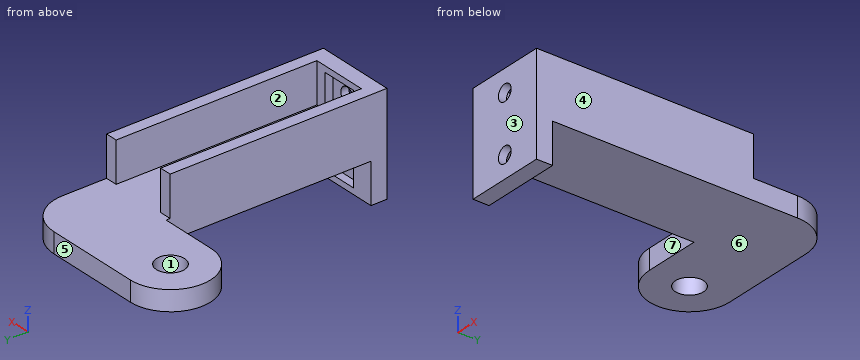
```python
from build123d import *

# Parameters (mm, degrees)
SKETCH1_R          = 1.75
AXLEHOLDER_DEPTH   = 2.5
SKETCH1_3_W        = 10
SKETCH1_3_H        = 2
BASE_DEPTH         = 7.5
BASE_DEPTH_BACK    = 5
SKETCH2_R          = 1
BOLTHOLES_DEPTH    = 3
SKETCH3_W          = 4.5
SKETCH3_H          = 4
NUTSLOTS_DEPTH     = 1
SKETCH4_W          = 1.5
SKETCH4_H          = 5
STIFFENERRIB_DEPTH = 25


with BuildPart() as part:
    # Sketch1 → AxleHolder (new body)
    with BuildSketch(Plane.XY):
        with BuildLine():
            Line((-12, 27.5), (-5, 27.5))
            Line((-5, 27.5), (-5, 0))
            Line((-5, 0), (5, 0))
            Line((5, 0), (5, 32.5))
            ThreePointArc((5, 32.5), (3.535533906, 36.035533906), (0, 37.5))
            Line((0, 37.5), (-12, 37.5))
            ThreePointArc((-12, 37.5), (-17, 32.5), (-12, 27.5))
        make_face()
        with Locations((-12, 32.5)):
            Circle(SKETCH1_R, mode=Mode.SUBTRACT)
    extrude(amount=AXLEHOLDER_DEPTH)

    # Sketch1<3> → Base (add, two sides)
    with BuildSketch(Plane.XY) as base_sk:
        with Locations((0, 1)):
            Rectangle(SKETCH1_3_W, SKETCH1_3_H)
    extrude(amount=BASE_DEPTH)
    extrude(base_sk.sketch, amount=-BASE_DEPTH_BACK)

    # Sketch2 → BoltHoles (cut, through all)
    with BuildSketch(Plane(origin=(0, 2, 0), x_dir=(1, 0, 0), z_dir=(0, 1, 0))):
        with Locations((0, 2.25)):
            Circle(SKETCH2_R)
        with Locations((0, -4.75)):
            Circle(SKETCH2_R)
    extrude(amount=-BOLTHOLES_DEPTH, mode=Mode.SUBTRACT)

    # Sketch3 → NutSlots (cut)
    with BuildSketch(Plane(origin=(0, 2, 0), x_dir=(1, 0, 0), z_dir=(0, 1, 0))):
        with Locations((0, -4.75)):
            Rectangle(SKETCH3_W, SKETCH3_H)
        with Locations((0, 2.25)):
            Rectangle(SKETCH3_W, SKETCH3_H)
    extrude(amount=-NUTSLOTS_DEPTH, mode=Mode.SUBTRACT)

    # Sketch4 → StiffenerRib (add)
    with BuildSketch(Plane(origin=(0, 2, 0), x_dir=(1, 0, 0), z_dir=(0, 1, 0))):
        with Locations((-4.25, -5)):
            Rectangle(SKETCH4_W, SKETCH4_H)
    stiffenerrib = extrude(amount=STIFFENERRIB_DEPTH)

    # StiffenerRib2: StiffenerRib across plane
    add(stiffenerrib.mirror(Plane(origin=(0, 0, 0), x_dir=(0, 0, 1), z_dir=(1, 0, 0))))


solid = part.part
```
For this review, take the finished solid that the model builds, in its own axes (mm). Face numbers are marked on the shaded views. A direction names the side the tool comes from. Round coordinates to 2 decimals unless told otherwise and drop trailing zeros. Write each loop counter-clockwise with the first axis right and the second up, starting at its lowest first coordinate (ties: lowest second). Pieces come first, ordered by that corner, then holes. Notation, with made-up numbers: (53, -23) -> (58, -23) arc R13 ccw to (58, 0) -> close; hole circle Ø7 at (56, 86). An arc over 180 degrees is marked (long way). One line per question, with ' | ' between items. Start each with the question number.
1) Add section D-D (y = 32). Write out the cut boundary in (x, z), and give its area (3 significant figures).
2) Add section B-B (y = 23). Write out the cut boundary in (x, z).
3) Add section A-A (z = 4.75). Write out the cut boundary in (x, y), and give its area (3 significant figures).
4) Wall thickness on line 1 along Z through (x, y) = (0, 0.8); line 2 along X through (y, z) = (0.35, 4.75); line 3 along X through (y, z) = (6.5, 3.75): over which ranges is each line inside the solid? List them lowest first.
5) For pin 1 Ø5.5 at (y, z) = (14.5, 5) entering from -X; pin 2 Ø6 at (y, z) = (31.5, 6) entering from +X; pin 3 Ø5 at (x, z) = (-10, -1) entering from -Y; pin 4 Ø3 at (x, z) = (0, -2.25) entering from +Y, all flat-tipped, find the tip position at first contact; note any pin that passes through.
6) Mouldability with a two-part tool opening along X and no side actions: class the marked faces 1, 2, 3 and 4 as +X half, -X half, draft (parallel to the pull), parting line (faces both ways), or undercut.
7) Add section C-C (x = -3). Write out the cut boundary in (y, z), and give its area (3 significant figures).
8) Machinability: for the marked faces 5, 6 and 7, which of the approach directions +Z, -Z, +X, -X, +Y, -Y give a long, thin tool a straight path to every point of the face, cutting with its end or side? Answer none if there is none.
Reported:
1) outline: (-16.97, 0) -> (-13.68, 0) -> (-13.68, 2.5) -> (-16.97, 2.5) -> close; (-10.32, 0) -> (5, 0) -> (5, 2.5) -> (-10.32, 2.5) -> close | area: 46.6 mm²
2) outline: (-5, 0) -> (5, 0) -> (5, 7.5) -> (3.5, 7.5) -> (3.5, 2.5) -> (-3.5, 2.5) -> (-3.5, 7.5) -> (-5, 7.5) -> close
3) outline: (-5, 0) -> (-1, 0) -> (-1, 1) -> (-2.25, 1) -> (-2.25, 2) -> (-3.5, 2) -> (-3.5, 27) -> (-5, 27) -> close; (1, 0) -> (5, 0) -> (5, 27) -> (3.5, 27) -> (3.5, 2) -> (2.25, 2) -> (2.25, 1) -> (1, 1) -> close | area: 88.5 mm²
4) line 1: z = -5 to -3.25, -1.25 to 3.75, 5.75 to 7.5 | line 2: x = -5 to -1, 1 to 5 | line 3: x = -5 to -3.5, 3.5 to 5
5) pin 1: stops at x = -5 | pin 2: passes through | pin 3: stops at y = 27.5 | pin 4: stops at y = 1
6) face 1: undercut | face 2: undercut | face 3: draft | face 4: +X half
7) outline: (0, -5) -> (2, -5) -> (2, 0) -> (37.5, 0) -> (37.5, 2.5) -> (2, 2.5) -> (2, 7.5) -> (0, 7.5) -> close | area: 114 mm²
8) face 5: +Z, -Z, +X, -X, +Y | face 6: -Z, +X, -X, +Y | face 7: +Z, -Z, -X, -Y
